Read the model definition and answer for the solid it produces. Units are mm, in the model's axes. A direction names the side the tool comes from. Coordinates: 2 decimals unless noted, no trailing zeros. Write each loop counter-clockwise with the first axis right and the second up, starting at its lowest first coordinate (ties: lowest second). Pieces come first, ordered by that corner, then holes. Notation, with made-up numbers: (1, 0) -> (52, 0) arc R29 ccw to (52, 25) -> close; hole circle Ø6 at (-24.75, 51). An arc over 180 degrees is marked (long way). Answer in a Markdown table with one row per item. Add a question column.
Item 1: Straight lines are drawn through the part: line 1 (Y direction, x = -51, z = 2.65); line 2 (Y direction, x = -63.5, z = 1.5); line 3 (Z direction, x = -27, y = 2). For each, find the intervals that lie inside material, in ascending order. Write a range as from..to.
Item 2: Given pin 1 Ø6 at (y, z) = (1, -4.5) entering from -X; pin 2 Ø2 at (x, z) = (-34.5, 20) entering from +Y; pin 3 Ø5 at (x, z) = (-43.5, -3) entering from +Y; pin 4 Ø5.5 at (y, z) = (9.5, 17) entering from +X, each flat-ended and moving along its own axis, determine where each tip first touches the part or whether it passes through.
Item 3: Section B-B on x = -76.5 is taken. Write down the section's boundary in (y, z), then the cut area to 3 significant figures.
Item 4: Which of the six approach directions +Z, -Z, +X, -X, +Y, -Y give full straight-line access (tool end or side, diameter ignored) to faces 4 (the face through (-29, 9, 8)), 5 (the face through (-41, 9, 8)), 6 (the face through (6, 14, -16)), 7 (the face through (-41, 7, 0))?
Item 5: Section A-A on y = -7 is taken. Write down the section's boundary in (x, z), then the cut area to 3 significant figures.
Item 6: Section C-C on x = -51 is taken. Write down the section's boundary in (y, z).
Item 7: For a pull along X with two mould halves and no side action, classify faces 1 (the face through (4, 9, -16)), 2 (the face through (-26.5, 9.07, 2.03)), 3 (the face through (6, 4, -16)) as +X half, -X half, draft (parallel to the pull), parting line (faces both ways), or undercut.
Item 8: Section D-D on z = -3.5 is taken. Write down the section's boundary in (x, y).
Autodesk Inventor part; units mm, degrees
ref_plane "YZ Plane" through (0, 0, 0) normal (1, 0, 0) x (0, 1, 0)
ref_plane "XZ Plane" through (0, 0, 0) normal (0, 1, 0) x (-1, 0, 0)
ref_plane "XY Plane" through (0, 0, 0) normal (0, 0, 1) x (1, 0, 0)
sketch "Sketch1" plane through (0, 0, 0) normal (0, 0, 1) x (1, 0, 0)
  line L0 (0, 0) -> (12, 0)
  line L1 (12, 0) -> (12, 18)
  line L2 (12, 18) -> (0, 18)
  line L3 (-29, 16.5) -> (-41, 16.5)
  line L4 (-41, 16.5) -> (-41, 1.5)
  line L5 (-41, 1.5) -> (-29, 1.5)
  line L6 (0, 18) -> (-29, 16.5)
  line L7 (0, 0) -> (-29, 1.5)
  circle A0 centre (-9, 9) radius 1.5
  dimension "d0" = 12
  dimension "d1" = 18
  dimension "d2" = 12
  dimension "d3" = 15
  dimension "d4" = 3
extrude "Extrusion1" add sketch "Sketch1" along normal blind 4
sketch "Sketch2" plane through (0, 0, 0) normal (0, 0, -1) x (-1, 0, 0)
  line L0 (0, 18) -> (29, 16.5)
  line L1 (0, 18) -> (-12, 18)
  line L2 (-12, 18) -> (-12, 0)
  line L3 (-12, 0) -> (0, 0)
  line L4 (0, 0) -> (0, 18)
  dimension "d11" = 12
  dimension "d7" = 12
  dimension "d8" = 18
extrude "Extrusion2" add sketch "Sketch2" along normal blind 11
sketch "Sketch3" plane through (0, 0, 4) normal (0, 0, 1) x (1, 0, 0)
  line L0 (-29, 16.5) -> (-41, 16.5)
  line L1 (-41, 16.5) -> (-29, 16.5)
  line L2 (-29, 16.5) -> (-29, 1.5)
  line L3 (-29, 1.5) -> (-41, 1.5)
  line L4 (-41, 1.5) -> (-41, 16.5)
  point P0 (0, 0)
  dimension "d11" = 12
  dimension "d12" = 15
extrude "Extrusion3" add sketch "Sketch3" along normal blind 9
sketch "Sketch4" plane through (0, 0, -11) normal (0, 0, -1) x (-1, 0, 0)
  line L0 (-4, 4) -> (-8, 4)
  line L1 (-8, 4) -> (-8, 14)
  line L2 (-8, 14) -> (-4, 14)
  line L3 (-4, 14) -> (-4, 4)
  point P0 (0, 0)
  dimension "d15" = 4
  dimension "d16" = 10
extrude "Extrusion4" add sketch "Sketch4" along normal blind 10
sketch "Sketch5" plane through (0, 0, 13) normal (0, 0, 1) x (1, 0, 0)
  line L0 (-33, 5.5) -> (-37, 5.5)
  line L1 (-37, 5.5) -> (-37, 12.5)
  line L2 (-37, 12.5) -> (-33, 12.5)
  line L3 (-33, 12.5) -> (-33, 5.5)
  point P0 (0, 0)
  dimension "d19" = 4
  dimension "d20" = 7
extrude "Extrusion5" add sketch "Sketch5" along normal blind 10
sketch "Sketch6" plane through (0, 0, 0) normal (0, 0, -1) x (-1, 0, 0)
  line L0 (41, 16.5) -> (41, 1.5)
  circle A0 centre (51, 9) radius 1.5
  line L1 (41, 16.5) -> (41, 1.5)
  line L2 (84, 1.5) -> (84, 16.5)
  line L3 (84, 16.5) -> (41, 16.5)
  line L4 (41, 16.5) -> (41, 1.5)
  line L5 (57, 1.5) -> (57, -23.5)
  line L6 (57, -23.5) -> (45, -23.5)
  line L7 (45, -23.5) -> (45, 1.5)
  line L8 (41, 1.5) -> (45, 1.5)
  line L9 (57, 1.5) -> (84, 1.5)
  point P0 (0, 0)
  dimension "d26" = 3
  dimension "d29" = 43
  dimension "d30" = 15
  dimension "d31" = 12
  dimension "d32" = 25
  dimension "d33" = 4
extrude "Extrusion7" add sketch "Sketch6" against normal blind 4
fillet "Fillet2" radius 4 4 edges at (-84, 16.5, 2) (-84, 1.5, 2) (-57, -23.5, 2) (-45, -23.5, 2)
sketch "Sketch7" plane through (0, 0, 4) normal (0, 0, 1) x (1, 0, 0)
  circle A0 centre (-63.5, 9) radius 1.5
  circle A1 centre (-76.5, 9) radius 1.5
  line L0 (-29, 16.5) -> (-41, 16.5)
  circle A2 centre (-51, 9) radius 1.5
  point P0 (0, 0)
  dimension "d39" = 3
  dimension "d40" = 3
  dimension "d41" = 7.5
  dimension "d42" = 7.5
  dimension "d43" = 12.5
  dimension "d44" = 13
extrude "Extrusion8" cut sketch "Sketch7" against normal through all contours A0 | A1
sketch "Sketch8" plane through (0, 0, 4) normal (0, 0, 1) x (1, 0, 0)
  circle A0 centre (-51, -7) radius 1.5
  line L0 (-45, -19.5) -> (-45, 1.5)
  circle A1 centre (-51, 9) radius 1.5
  point P0 (0, 0)
  dimension "d47" = 3
  dimension "d48" = 6
  dimension "d49" = 16
extrude "Extrusion9" cut sketch "Sketch8" against normal through all contours A0
sketch "Sketch9" plane through (0, 0, 4) normal (0, 0, 1) x (1, 0, 0)
  point P0 (0, 0)
sketch "Sketch10" plane through (0, 0, 4) normal (0, 0, 1) x (1, 0, 0)
  circle A0 centre (-25, 9) radius 1.5
  line L0 (-29, 16.5) -> (-41, 16.5)
  circle A1 centre (-9, 9) radius 1.5
  point P0 (0, 0)
  dimension "d52" = 3
  dimension "d53" = 7.5
  dimension "d54" = 16
extrude "Extrusion10" cut sketch "Sketch10" against normal through all contours A0
properties part number "Mounting Bracket 3of4 - Copy"
Results below:
| question | item | result |
|---|---|---|
| 1 | line 1 | y = -23.5..-8.5, -5.5..7.5, 10.5..16.5 |
| 1 | line 2 | y = 1.5..7.5, 10.5..16.5 |
| 1 | line 3 | z = 0..4 |
| 2 | pin 1 | stops at x = 0 |
| 2 | pin 2 | stops at y = 12.5 |
| 2 | pin 3 | passes through |
| 2 | pin 4 | stops at x = -33 |
| 3 | outline | (1.5, 0) -> (7.5, 0) -> (7.5, 4) -> (1.5, 4) -> close; (10.5, 0) -> (16.5, 0) -> (16.5, 4) -> (10.5, 4) -> close |
| 3 | area | 48.0 mm2 |
| 4 | face 4 | +Z, +X, +Y, -Y |
| 4 | face 5 | +Z, -X, +Y, -Y |
| 4 | face 6 | -Z, +X, -X, +Y |
| 4 | face 7 | -Z, -X, +Y, -Y |
| 5 | outline | (-57, 0) -> (-52.5, 0) -> (-52.5, 4) -> (-57, 4) -> close; (-49.5, 0) -> (-45, 0) -> (-45, 4) -> (-49.5, 4) -> close |
| 5 | area | 36.0 mm2 |
| 6 | outline | (-23.5, 0) -> (-8.5, 0) -> (-8.5, 4) -> (-23.5, 4) -> close; (-5.5, 0) -> (7.5, 0) -> (7.5, 4) -> (-5.5, 4) -> close; (10.5, 0) -> (16.5, 0) -> (16.5, 4) -> (10.5, 4) -> close |
| 7 | face 1 | -X half |
| 7 | face 2 | undercut |
| 7 | face 3 | draft |
| 8 | outline | (0, 0) -> (12, 0) -> (12, 18) -> (0, 18) -> close |
